Check sheet for the drawn part. Datum: minimum x, y, z corner. Units: mm. A direction names the side the tool comes from. Coordinates: 2 decimals unless noted, no trailing zeros. Order: outer loops, then holes, each group sorted by start corner. A loop starts at its lowest first (then second) coordinate and runs counter-clockwise, first axis right, second up.
1. Set-up check for the marked faces 1, 2 and 3: record each of +Z, -Z, +X, -X, +Y, -Y from which the full face is reachable in a straight line by a thin tool's end or side.
2. Cross-section at A-A (y = 2.5). Enter the section's corners in (x, z) (3 decimals), then the cut area to 3 significant figures.
3. Thickness scan on line 1 (X direction, y = 31, z = 36.5); line 2 (Y direction, x = 63.5, z = 11.5); line 3 (Z direction, x = 71, y = 5) (3 decimals). Record the ranges inside material, lowest first.
4. Cross-section at B-B (x = 72.5). Enter the section's corners in (y, z) (3 decimals), then the cut area to 3 significant figures.
5. Gauge pin test, flat ends, axial feed: pin 1 Ø4 at (y, z) = (6, 9.5) entering from +X; pin 2 Ø5 at (x, z) = (84, 8.5) entering from +Y; pin 3 Ø5 at (x, z) = (111.5, 34.5) entering from -Y; pin 4 Ø14 at (x, y) = (33, 4.5) entering from +Z (3 decimals). Record the tip position at first contact, or that the pin passes through.
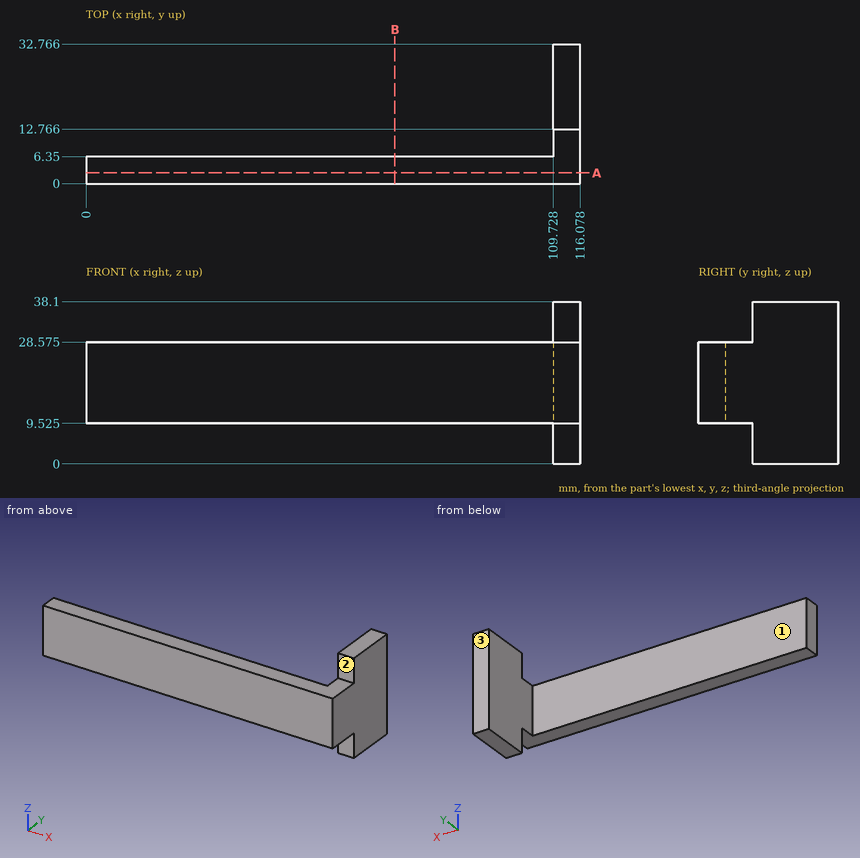
Data:
1. face 1: +Z, -Z, -X, +Y
1. face 2: +Z, +X, -X, -Y
1. face 3: +Z, -Z, +X, -X, +Y
2. outline: (0, 9.525) - (116.078, 9.525) - (116.078, 28.575) - (0, 28.575) - close
2. area: 2,210 mm2
3. line 1: x = 109.73 to 116.08
3. line 2: y = 0 to 6.35
3. line 3: z = 9.525 to 28.575
4. outline: (0, 9.525) - (6.35, 9.525) - (6.35, 28.575) - (0, 28.575) - close
4. area: 121 mm2
5. pin 1: stops at x = 116.08
5. pin 2: stops at y = 6.35
5. pin 3: stops at y = 12.77
5. pin 4: stops at z = 28.575
